Source: CAD feature listing. Evaluate the final solid. Frame: model axes, mm. Round coordinates to 2 decimals unless told otherwise and drop trailing zeros. Loops run counter-clockwise (first coordinate to the right, second up) from the corner with the lowest first, then second, coordinate; pieces in that order, holes last. Notation, with made-up numbers: M 22.25,75.25 L 33.25,75.25 A20 ccw 33.25,79.25 Z; hole C -38,-3.75 d8. An arc over 180 degrees is marked long. Answer as a JSON object with one key per item and string values.
from build123d import *

# Parameters (mm, degrees)
SKETCH1_R           = 2
BOSS_EXTRUDE1_DEPTH = 4.5
CHAMFER1_SIZE       = 3
CHAMFER2_SIZE       = 3


with BuildPart() as part:
    # Sketch1 → Boss-Extrude1 (new body)
    with BuildSketch(Plane.XY):
        with BuildLine():
            Line((-12, 6), (12, 6))
            ThreePointArc((12, 6), (18, 0), (12, -6))
            Line((12, -6), (-12, -6))
            ThreePointArc((-12, -6), (-18, 0), (-12, 6))
        make_face()
        with Locations((-12, 0)):
            Circle(SKETCH1_R, mode=Mode.SUBTRACT)
        with Locations((12, 0)):
            Circle(SKETCH1_R, mode=Mode.SUBTRACT)
    extrude(amount=BOSS_EXTRUDE1_DEPTH)

    # Chamfer1
    chamfer1_edges = [part.edges().sort_by_distance(p)[0] for p in [
        (10, 0, 0),
    ]]
    chamfer(chamfer1_edges, length=CHAMFER1_SIZE)

    # Chamfer2
    chamfer2_edges = [part.edges().sort_by_distance(p)[0] for p in [
        (-14, 0, 4.5),
    ]]
    chamfer(chamfer2_edges, length=CHAMFER2_SIZE)


solid = part.part
Item 1: Section B-B on z = 4.05. Return the cut outline in (x, y), then the cut area to 3 significant figures.
Answer sheet:
{"outline": "M -12,-6 L 12,-6 A6 ccw 12,6 L -12,6 A6 ccw Z; hole C -12,0 d9.1; hole C 12,0 d4", "area": "323 mm²"}
Item 2: Pull-direction query (Y, two-part tool) for faces 1 (the flat face through (-4, 0, 0)), 2 (the cylindrical face through (-13.6, -1.2, 0.7)), 3 (the flat face through (0, 6, 2)); classes: pulls with the +Y half, pulls with the -Y half, needs draft (parallel to the pull), parting line crosses it, or undercut.
Answer sheet:
{"face 1": "needs draft", "face 2": "undercut", "face 3": "pulls with the +Y half"}
Item 3: Line query: probe 1 along X at (y, z) = (0.25, 4.1); probe 2 along Y at (x, z) = (12, 4.1); probe 3 along X at (y, z) = (-2, 2.45). Output: solid intervals per line, ascending. Write a range as from..to.
Answer sheet:
{"probe 1": "x = -17.99..-16.59, -7.41..10.02, 13.98..17.99", "probe 2": "y = -6..-2, 2..6", "probe 3": "x = -17.66..-14.17, -9.83..10.42, 13.58..17.66"}
Item 4: Contact query for flat-ended pins moving along their axis: pin 1 Ø1.5 at (y, z) = (3.5, 1) entering from -X; pin 2 Ø1.5 at (y, z) = (-1, 2) entering from +X; pin 3 Ø1 at (y, z) = (-2, 3) entering from +X. Output: stop coordinate, or through.
Answer sheet:
{"pin 1": "stops at x = -17.33", "pin 2": "stops at x = 17.99", "pin 3": "stops at x = 17.81"}
Item 5: Section A-A on y = 0. Return the cut outline in (x, z).
Answer sheet:
{"outline": "M -18,0 L -14,0 L -14,1.5 L -17,4.5 L -18,4.5 Z; M -10,0 L 7,0 L 10,3 L 10,4.5 L -7,4.5 L -10,1.5 Z; M 14,3 L 17,0 L 18,0 L 18,4.5 L 14,4.5 Z"}
